from build123d import *

# Parameters (mm, degrees)
SKETCH1_R           = 2.25
BOSS_EXTRUDE1_DEPTH = 2.5
SKETCH3_W           = 50
SKETCH3_H           = 5
BOSS_EXTRUDE2_DEPTH = 32
SKETCH7_R           = 5
CUT_EXTRUDE3_DEPTH  = 7
SKETCH5_R           = 7.95
SKETCH5_W           = 10
SKETCH5_H           = 16
CUT_EXTRUDE1_DEPTH  = 7
SKETCH8_W           = 50
SKETCH8_H           = 18
CUT_EXTRUDE4_DEPTH  = 46.265881191
SKETCH9_W           = 50
SKETCH9_H           = 2.5
BOSS_EXTRUDE3_DEPTH = 50
SKETCH10_R          = 2.25
CUT_EXTRUDE5_DEPTH  = 81.925892025
FILLET1_R           = 5


with BuildPart() as part:
    # Sketch1 → Boss-Extrude1 (new body)
    with BuildSketch(Plane(origin=(0, 0, 0), x_dir=(1, 0, 0), z_dir=(0, 1, 0))):
        Polygon((-12, -20), (12, -20), (12, -2), (16, -2), (16, -20), (25, -20), (25, 20), (-25, 20), (-25, -20), (-16, -20), (-16, -2), (-12, -2), align=None)
        with Locations(Location((-16, 16, 0), (0, 0, 270))):
            Circle(SKETCH1_R, mode=Mode.SUBTRACT)
        with Locations(Location((-16, 8, 0), (0, 0, 270))):
            Circle(SKETCH1_R, mode=Mode.SUBTRACT)
        with Locations(Location((16, 16, 0), (0, 0, 270))):
            Circle(SKETCH1_R, mode=Mode.SUBTRACT)
        with Locations(Location((16, 8, 0), (0, 0, 270))):
            Circle(SKETCH1_R, mode=Mode.SUBTRACT)
    extrude(amount=BOSS_EXTRUDE1_DEPTH)

    # Sketch3 → Boss-Extrude2 (add)
    with BuildSketch(Plane(origin=(0, 2.5, 0), x_dir=(1, 0, 0), z_dir=(0, 1, 0))):
        with Locations((0, 1.5)):
            Rectangle(SKETCH3_W, SKETCH3_H)
    extrude(amount=BOSS_EXTRUDE2_DEPTH)

    # Sketch7 → Cut-Extrude3 (cut)
    with BuildSketch(Plane(origin=(0, 2.5, 0), x_dir=(1, 0, 0), z_dir=(0, 1, 0))):
        with Locations(Location((0, 9, 0), (0, 0, 270))):
            Circle(SKETCH7_R)
    extrude(amount=-CUT_EXTRUDE3_DEPTH, mode=Mode.SUBTRACT)

    # Sketch5 → Cut-Extrude1 (cut)
    with BuildSketch(Plane.XY.offset(1)):
        with Locations((-13, 23.5)):
            Circle(SKETCH5_R)
        with Locations((13, 23.5)):
            Circle(SKETCH5_R)
        with Locations((0, 10.494306312)):
            Rectangle(SKETCH5_W, SKETCH5_H)
    extrude(amount=-CUT_EXTRUDE1_DEPTH, mode=Mode.SUBTRACT)

    # Sketch8 → Cut-Extrude4 (cut, through all)
    with BuildSketch(Plane(origin=(0, 2.5, 0), x_dir=(1, 0, 0), z_dir=(0, 1, 0))):
        with Locations((0, -11)):
            Rectangle(SKETCH8_W, SKETCH8_H)
    extrude(amount=-CUT_EXTRUDE4_DEPTH, mode=Mode.SUBTRACT)

    # Sketch9 → Boss-Extrude3 (add)
    with BuildSketch(Plane(origin=(0, 0, -20), x_dir=(-1, 0, 0), z_dir=(0, 0, -1))):
        with Locations((0, 1.25)):
            Rectangle(SKETCH9_W, SKETCH9_H)
    extrude(amount=BOSS_EXTRUDE3_DEPTH)

    # Sketch10 → Cut-Extrude5 (cut, through all)
    with BuildSketch(Plane(origin=(0, 2.5, 0), x_dir=(1, 0, 0), z_dir=(0, 1, 0))):
        with Locations(Location((-16, 16, 0), (0, 0, 270))):
            Circle(SKETCH10_R)
        with Locations(Location((-16, 24, 0), (0, 0, 270))):
            Circle(SKETCH10_R)
        with Locations(Location((-16, 32, 0), (0, 0, 270))):
            Circle(SKETCH10_R)
        with Locations(Location((-16, 40, 0), (0, 0, 270))):
            Circle(SKETCH10_R)
        with Locations(Location((16, 40, 0), (0, 0, 90))):
            Circle(SKETCH10_R)
        with Locations(Location((16, 32, 0), (0, 0, 90))):
            Circle(SKETCH10_R)
        with Locations(Location((16, 24, 0), (0, 0, 90))):
            Circle(SKETCH10_R)
    extrude(amount=-CUT_EXTRUDE5_DEPTH, mode=Mode.SUBTRACT)

    # Fillet1
    fillet1_edges = [part.edges().sort_by_distance(p)[0] for p in [
        (25, 1.25, -70),
        (-25, 1.25, -70),
        (-25, 34.5, -1.5),
        (25, 34.5, -1.5),
    ]]
    fillet(fillet1_edges, radius=FILLET1_R)


solid = part.part
Here's how the part is built. I have some questions about the finished solid (model axes, mm). A direction names the side the tool comes from. Coordinates: 2 decimals unless noted, no trailing zeros. Order: outer loops, then holes, each group sorted by start corner. A loop starts at its lowest first (then second) coordinate and runs counter-clockwise, first axis right, second up. Notation, with made-up numbers: M -6,59.25 L 18,59.25 A31 ccw 18,86.25 Z; hole C 85.5,-5 d10. An arc over 180 degrees is marked long. Answer as CSV lines item,"result". Start each with the question number.
1. For pin 1 (3.5 mm diameter, centred on x = 16, z = -24, fed in from +Y); pin 2 (12 mm diameter, centred on y = 14.5, z = -9, fed in from +X); pin 3 (9.5 mm diameter, centred on x = -1, y = 24, fed in from -Z); pin 4 (5 mm diameter, centred on x = 16, z = -8, fed in from +Y), each with a flat end and sliding along its axis, tell me the tip position at first contact or that it passes through.
2. I want a section at A-A, the plane y = 3.5. Write out the boundary of the cut face in (x, z), and give its area (3 significant figures).
3. I want a section at D-D, the plane z = -32. Write out the boundary of the cut face in (x, y).
4. I want a section at B-B, the plane z = -2.5. Write out the boundary of the cut face in (x, y).
5. On a 3-axis mill with a long thin cutter (end or side, diameter ignored), from which of +Z, -Z, +X, -X, +Y, -Y can I reach the whole of each face in a straight line? I mean faces 5 (the flat face through (25, 2, -16)), 6 (the flat face through (0, 2.5, -37)), 7 (the flat face through (0, 2.494, -2)). Say none if no direction works.
6. We'd pull the mould along X, two halves only. Please class faces 1 (the cylindrical face through (16.86, 1.27, -34.08)), 2 (the cylindrical face through (23.57, 33, -1.54)), 3 (the flat face through (0, 34.5, -2)), 4 (the cylindrical face through (-23, 1, -69)): released by +X, released by -X, zero draft, split by the parting line, or undercut.
7. I need wall thicknesses on line 1 (X direction, y = 1, z = -8); line 2 (X direction, y = 19.5, z = -2); line 3 (Y direction, x = -13, z = -2.65). Which ranges of each line are inside material? Lowest first, please. Write a range as [from, to].
8. I want a section at C-C, the plane x = 3. Count the separate pieces of the cut face and the enclosed holes in it, and give its area (3 significant figures).
Recorded:
1,pin 1,"passes through"
1,pin 2,"stops at x = 25"
1,pin 3,"stops at z = -4"
1,pin 4,"stops at y = 2.5"
2,outline,"M -25,-4 L -5,-4 L -5,1 L -25,1 Z; M 5,-4 L 25,-4 L 25,1 L 5,1 Z"
2,area,"200 mm2"
3,outline,"M -25,0 L -18.25,0 L -18.25,2.5 L -25,2.5 Z; M -13.75,0 L 13.75,0 L 13.75,2.5 L -13.75,2.5 Z; M 18.25,0 L 25,0 L 25,2.5 L 18.25,2.5 Z"
4,outline,"M -25,0 L 25,0 L 25,29.5 A5 ccw 20,34.5 L -20,34.5 A5 ccw -25,29.5 Z; hole C -13,23.5 d15.9; hole M -5,2.49 L 5,2.49 L 5,18.49 L -5,18.49 Z; hole C 13,23.5 d15.9"
5,face 5,"+Z, -Z, +X, +Y, -Y"
5,face 6,"-Z, +X, -X, +Y"
5,face 7,"+Z, -Z"
6,face 1,"undercut"
6,face 2,"released by +X"
6,face 3,"zero draft"
6,face 4,"released by -X"
7,line 1,"x = [-25, -18.25], [-13.75, -4.9], [4.9, 13.75], [18.25, 25]"
7,line 2,"x = [-25, -19.87], [-6.13, 6.13], [19.87, 25]"
7,line 3,"y = [0, 15.55], [31.45, 34.5]"
8,separate pieces,"3"
8,enclosed holes,"0"
8,area,"240 mm2"
